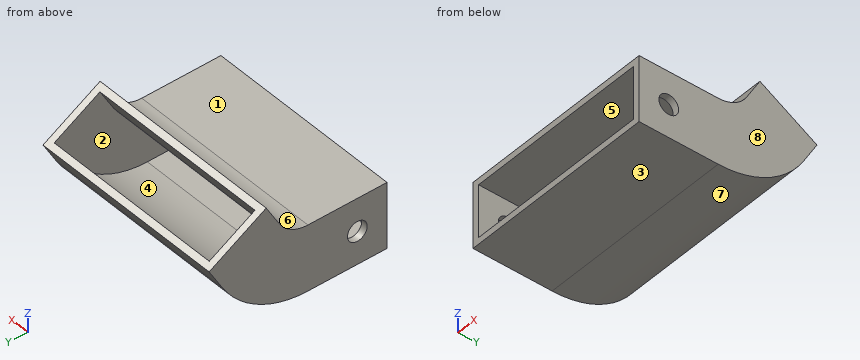
from build123d import *

# Parameters (mm, degrees)
SKETCH1_W           = 30
SKETCH1_H           = 10
SKETCH1_W_2         = 28
SKETCH1_H_2         = 8
BOSS_EXTRUDE1_DEPTH = 12
SWEEP1_START        = -15
SWEEP1_DEPTH        = 30
SWEEP1_2_DEPTH      = 1
SWEEP1_START_2      = 14
SWEEP1_3_DEPTH      = 1
SKETCH4_W           = 30
SKETCH4_H           = 10
SKETCH4_W_2         = 28
SKETCH4_H_2         = 8
BOSS_EXTRUDE2_DEPTH = 4
SKETCH7_R           = 1.5
CUT_EXTRUDE1_DEPTH  = 42.817367132


# Read off the part's stored shape, not the designer's step: Sweep1
with BuildPart() as part:
    # Sketch1 → Boss-Extrude1 (new body)
    with BuildSketch(Plane(origin=(0, 0, 0), x_dir=(1, 0, 0), z_dir=(0, 1, 0))):
        Rectangle(SKETCH1_W, SKETCH1_H)
        Rectangle(SKETCH1_W_2, SKETCH1_H_2, mode=Mode.SUBTRACT)
    extrude(amount=BOSS_EXTRUDE1_DEPTH)

    # Sweep1 outline → Sweep1 (add)
    with BuildSketch(Plane.YZ.offset(SWEEP1_START)):
        with BuildLine():
            ThreePointArc((16.330127019, 7.5), (14.5, 5.669872981), (12, 5))
            Line((12, 5), (12, 4))
            ThreePointArc((12, 4), (15, 4.803847577), (17.196152423, 7))
            Line((17.196152423, 7), (16.330127019, 7.5))
        make_face()
        with BuildLine():
            ThreePointArc((24.124355653, 3), (19, -2.124355653), (12, -4))
            Line((12, -4), (12, -5))
            ThreePointArc((12, -5), (19.5, -2.990381057), (24.990381057, 2.5))
            Line((24.990381057, 2.5), (24.124355653, 3))
        make_face()
    extrude(amount=SWEEP1_DEPTH)

    # Sweep1 2 outline → Sweep1 2 (add)
    with BuildSketch(Plane.YZ.offset(SWEEP1_START)):
        with BuildLine():
            ThreePointArc((17.196152423, 7), (15, 4.803847577), (12, 4))
            Line((12, 4), (12, -4))
            ThreePointArc((12, -4), (19, -2.124355653), (24.124355653, 3))
            Line((24.124355653, 3), (17.196152423, 7))
        make_face()
    extrude(amount=SWEEP1_2_DEPTH)

    # Sweep1 3 outline → Sweep1 3 (add)
    with BuildSketch(Plane.YZ.offset(SWEEP1_START_2)):
        with BuildLine():
            ThreePointArc((17.196152423, 7), (15, 4.803847577), (12, 4))
            Line((12, 4), (12, -4))
            ThreePointArc((12, -4), (19, -2.124355653), (24.124355653, 3))
            Line((24.124355653, 3), (17.196152423, 7))
        make_face()
    extrude(amount=SWEEP1_3_DEPTH)

    # Sketch4 → Boss-Extrude2 (add)
    with BuildSketch(Plane(origin=(0, 7.330127019, 12.696152423), x_dir=(1, 0, 0), z_dir=(0, 0.4999999999999947, 0.8660254037844418))):
        with Locations((0, 15.392304845)):
            Rectangle(SKETCH4_W, SKETCH4_H)
        with Locations((0, 15.392304845)):
            Rectangle(SKETCH4_W_2, SKETCH4_H_2, mode=Mode.SUBTRACT)
    extrude(amount=BOSS_EXTRUDE2_DEPTH)

    # Sketch7 → Cut-Extrude1 (cut, through all)
    with BuildSketch(Plane.ZY.offset(15)):
        with Locations((0, 4.5)):
            Circle(SKETCH7_R)
    extrude(amount=-CUT_EXTRUDE1_DEPTH, mode=Mode.SUBTRACT)


solid = part.part
Here's how the part is built. I have some questions about the finished solid (model axes, mm). Face numbers are marked on the shaded views. A direction names the side the tool comes from. Round coordinates to 2 decimals unless told otherwise and drop trailing zeros. Loops run counter-clockwise (first coordinate to the right, second up) from the corner with the lowest first, then second, coordinate; pieces in that order, holes last. Notation, with made-up numbers: (79, 72.25) - (94, 72.25) arc R18 ccw to (94, 103.25) - close; hole circle Ø10 at (51.25, 56). An arc over 180 degrees is marked (long way). One line per question, with ' | ' between items. Start each with the question number.
Q1. We'd pull the mould along Z, two halves only. Please class the marked faces 5, 6, 7 and 8: +Z half, -Z half, draft (parallel to the pull), parting line (faces both ways), or undercut.
Q2. I want a section at A-A (x = -7.5). Write out the boundary of the cut face in (y, z).
Q3. Please list where these lines run through material, in increasing order: line 1 (Z direction, x = -3, y = 11); line 2 (X direction, y = 17, z = 6.25); line 3 (Y direction, x = -14.4, z = 0). Write a range as [from, to].
Q4. I want a section at C-C (z = 0). Write out the boundary of the cut face in (x, y), then the cut area to 3 significant figures.
Q5. I want a section at D-D (y = 20.5). Write out the boundary of the cut face in (x, z).
Q6. I want a section at B-B (y = 4.5). Write out the boundary of the cut face in (x, z), then the cut area to 3 significant figures.
Q7. For the marked faces 1, 2, 3 and 4, which set-ups out of +Z, -Z, +X, -X, +Y, -Y let a thin tool reach every point of the face, with its end or its side?
Q8. Will these pins go through, and if not, where does the flat tip stop? pin 1 (1.5 mm diameter, centred on x = 1.5, z = -1.5, fed in from +Y); pin 2 (4 mm diameter, centred on x = -8.5, y = 18.5, fed in from +Z); pin 3 (8 mm diameter, centred on x = -5.5, z = 9.5, fed in from -Y); pin 4 (2.5 mm diameter, centred on y = 4.5, z = 0, fed in from +X).
Response values:
1) face 5: undercut | face 6: +Z half | face 7: -Z half | face 8: draft
2) outline: (0, -5) - (12, -5) arc R15 ccw to (24.99, 2.5) - (26.99, 5.96) - (26.12, 6.46) - (24.12, 3) arc R14 cw to (12, -4) - (0, -4) - close; (0, 4) - (12, 4) arc R6 ccw to (17.2, 7) - (19.2, 10.46) - (18.33, 10.96) - (16.33, 7.5) arc R5 cw to (12, 5) - (0, 5) - close
3) line 1: z = [-5, -4], [4, 5] | line 2: x = [-15, -14], [14, 15] | line 3: y = [0, 3], [6, 23.18]
4) outline: (-15, 0) - (-14, 0) - (-14, 3) - (-15, 3) - close; (-15, 6) - (-14, 6) - (-14, 21.8) - (14, 21.8) - (14, 6) - (15, 6) - (15, 23.18) - (-15, 23.18) - close; (14, 0) - (15, 0) - (15, 3) - (14, 3) - close | area: 79.1 mm²
5) outline: (-15, -2.36) - (15, -2.36) - (15, 9.71) - (14, 9.71) - (14, -1.12) - (-14, -1.12) - (-14, 9.71) - (-15, 9.71) - close
6) outline: (-15, -5) - (15, -5) - (15, -1.5) - (14, -1.5) - (14, -4) - (-14, -4) - (-14, -1.5) - (-15, -1.5) - close; (-15, 1.5) - (-14, 1.5) - (-14, 4) - (14, 4) - (14, 1.5) - (15, 1.5) - (15, 5) - (-15, 5) - close | area: 70.0 mm²
7) face 1: +Z, +X, -X, -Y | face 2: none | face 3: -Z, +X, -X, +Y, -Y | face 4: -Y
8) pin 1: stops at y = 22.46 | pin 2: stops at z = 10.96 | pin 3: stops at y = 14.18 | pin 4: passes through
